Read the model definition and answer for the solid it produces. Units are mm, in the model's axes. Face numbers are marked on the shaded views. A direction names the side the tool comes from. Coordinates: 2 decimals unless noted, no trailing zeros. Order: outer loops, then holes, each group sorted by start corner. A loop starts at its lowest first (then second) coordinate and runs counter-clockwise, first axis right, second up. Notation, with made-up numbers: M 26,21.5 L 33,21.5 A10 ccw 33,29.5 Z; hole C 10,49 d7. An arc over 180 degrees is marked long. Put each result on its own line as item: value.
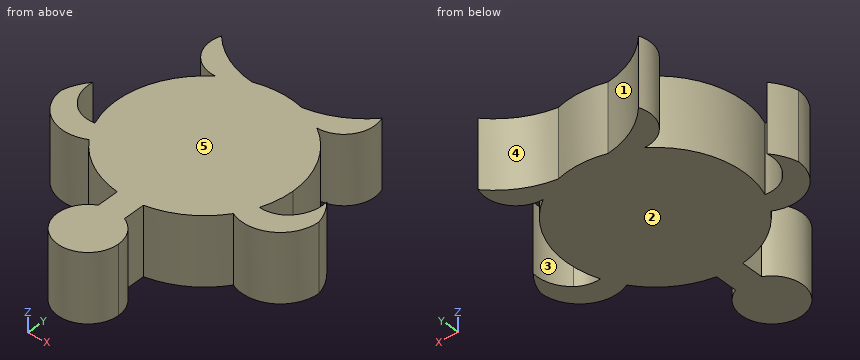
from build123d import *

# Parameters (mm, degrees)
F1_DEPTH = 2


with BuildPart() as f1:
    # F0 (on Top) → F1 (new body)
    with BuildSketch(Plane.XY):
        with BuildLine():
            ThreePointArc((-1.484384, 2.124211), (-1.120709, 2.336596), (-0.727436, 2.487269))
            ThreePointArc((-0.727436, 2.487269), (-1.616601, 2.768638), (-2.351094, 3.343359))
            ThreePointArc((-2.351094, 3.343359), (-2.243244, 2.502379), (-1.484384, 2.124211))
        make_face()
        with BuildLine():
            ThreePointArc((-2.113658, -1.499373), (-2.279864, -1.232027), (-2.412428, -0.9465))
            ThreePointArc((-2.412428, -0.9465), (-2.750971, -0.923594), (-3.055104, -0.773129))
            ThreePointArc((-3.055104, -0.773129), (-3.36643, -0.345932), (-3.426473, 0.17925))
            ThreePointArc((-3.426473, 0.17925), (-3.640466, -0.140011), (-3.772722, -0.500882))
            ThreePointArc((-3.772722, -0.500882), (-3.219918, -1.459931), (-2.113658, -1.499373))
        make_face()
        with BuildLine():
            ThreePointArc((3.055104, -0.773129), (2.750971, -0.923594), (2.412428, -0.9465))
            ThreePointArc((2.412428, -0.9465), (2.279864, -1.232027), (2.113658, -1.499373))
            ThreePointArc((2.113658, -1.499373), (3.219918, -1.459931), (3.772722, -0.500882))
            ThreePointArc((3.772722, -0.500882), (3.640466, -0.140011), (3.426473, 0.17925))
            ThreePointArc((3.426473, 0.17925), (3.36643, -0.345932), (3.055104, -0.773129))
        make_face()
        with BuildLine():
            ThreePointArc((0.892009, -4.021506), (0.754487, -3.54566), (0.384325, -3.216537))
            ThreePointArc((0.384325, -3.216537), (0, -3.129497), (-0.384325, -3.216537))
            ThreePointArc((-0.384325, -3.216537), (-0.475846, -4.775993), (0.892009, -4.021506))
        make_face()
        with BuildLine():
            ThreePointArc((2.591461, 0), (2.298085, 1.197695), (1.484384, 2.124211))
            ThreePointArc((1.484384, 2.124211), (1.120709, 2.336596), (0.727436, 2.487269))
            ThreePointArc((0.727436, 2.487269), (0, 2.591461), (-0.727436, 2.487269))
            ThreePointArc((-0.727436, 2.487269), (-1.120709, 2.336596), (-1.484384, 2.124211))
            ThreePointArc((-1.484384, 2.124211), (-2.480645, 0.749711), (-2.412428, -0.9465))
            ThreePointArc((-2.412428, -0.9465), (-2.276223, -1.230181), (-2.111146, -1.498092))
            ThreePointArc((-2.111146, -1.498092), (-2.112401, -1.498733), (-2.113658, -1.499373))
            ThreePointArc((-2.113658, -1.499373), (-1.357461, -2.20748), (-0.384325, -2.562804))
            ThreePointArc((-0.384325, -2.562804), (0, -2.591461), (0.384325, -2.562804))
            ThreePointArc((0.384325, -2.562804), (1.357461, -2.20748), (2.113658, -1.499373))
            ThreePointArc((2.113658, -1.499373), (2.279864, -1.232027), (2.412428, -0.9465))
            ThreePointArc((2.412428, -0.9465), (2.546309, -0.481642), (2.591461, 0))
        make_face()
        with BuildLine():
            ThreePointArc((0.727436, 2.487269), (1.120709, 2.336596), (1.484384, 2.124211))
            ThreePointArc((1.484384, 2.124211), (2.243244, 2.502379), (2.351094, 3.343359))
            ThreePointArc((2.351094, 3.343359), (1.616601, 2.768638), (0.727436, 2.487269))
        make_face()
        with BuildLine():
            Line((0.384325, -3.216537), (0.384325, -2.562804))
            ThreePointArc((0.384325, -2.562804), (0, -2.591461), (-0.384325, -2.562804))
            Line((-0.384325, -2.562804), (-0.384325, -3.216537))
            ThreePointArc((-0.384325, -3.216537), (0, -3.129497), (0.384325, -3.216537))
        make_face()
        with BuildLine():
            ThreePointArc((-2.111146, -1.498092), (-2.276223, -1.230181), (-2.412428, -0.9465))
            ThreePointArc((-2.412428, -0.9465), (-2.279864, -1.232027), (-2.113658, -1.499373))
            ThreePointArc((-2.113658, -1.499373), (-2.112401, -1.498733), (-2.111146, -1.498092))
        make_face()
    extrude(amount=F1_DEPTH)


solid = f1.part
Q1. Consider line 1 along Y through (x, z) = (0, 0.6); line 2 along X through (y, z) = (-0.5, 1.3); line 3 along Y through (x, z) = (-1.75, 1.6). Determine where each line is inside the solid, lowest interval first.
Answers below:
line 1: y = -4.91 to 2.59
line 2: x = -3.77 to -3.29, -2.54 to 2.54, 3.29 to 3.77
line 3: y = -1.91 to 1.91, 2.16 to 2.84
Q2. A tool of negligible diameter and unlimited length cuts with its end or side. For the marked faces 1, 2 and 3, from which of +Z, -Z, +X, -X, +Y, -Y can it reach the whole face along a straight path? Write none if from no direction.
Answers below:
face 1: +Z, -Z, +Y
face 2: -Z, +X, -X, +Y, -Y
face 3: +Z, -Z
Q3. Given pin 1 (0.7 mm diameter, centred on y = -3, z = 1, fed in from -X), flat-ended and moving along its own axis, determine where the tip first touches the part or whether it passes through.
Answers below:
pin 1: stops at x = -0.59
Q4. Find section C-C on x = 0. Write down the section's boundary in (y, z).
Answers below:
outline: M -4.91,0 L 2.59,0 L 2.59,2 L -4.91,2 Z
Q5. For a pull along X with two mould halves and no side action, classify the marked faces 4 and 5 as +X half, -X half, draft (parallel to the pull), parting line (faces both ways), or undercut.
Answers below:
face 4: undercut
face 5: draft
Q6. Find section A-A on y = 2.75. Write down the section's boundary in (x, z), plus the area to 3 significant figures.
Answers below:
outline: M -2.37,0 L -1.58,0 L -1.58,2 L -2.37,2 Z; M 1.58,0 L 2.37,0 L 2.37,2 L 1.58,2 Z
area: 3.15 mm^2
Q7. Find section B-B on z = 0.55. Write down the section's boundary in (x, y), plus the area to 3 significant figures.
Answers below:
outline: M -3.77,-0.5 A1.14 ccw -2.11,-1.5 A2.59 ccw -0.38,-2.56 L -0.38,-3.22 A0.89 ccw long 0.89,-4.02 A0.89 ccw 0.38,-3.22 L 0.38,-2.56 A2.59 ccw 2.11,-1.5 A1.14 ccw 3.77,-0.5 A1.61 ccw 3.43,0.18 A1.04 cw 3.06,-0.77 A0.87 cw 2.41,-0.95 A2.59 ccw 2.59,0 A2.59 ccw 1.48,2.12 A0.9 ccw 2.35,3.34 A2.62 cw 0.73,2.49 A2.59 ccw -0.73,2.49 A2.62 cw -2.35,3.34 A0.9 ccw -1.48,2.12 A2.59 ccw -2.41,-0.95 A0.87 cw -3.06,-0.77 A1.04 cw -3.43,0.18 A1.61 ccw Z
area: 28.1 mm^2
Q8. Find section D-D on y = -1.25. Write down the section's boundary in (x, z), plus the area to 3 significant figures.
Answers below:
outline: M -3.48,0 L 3.48,0 L 3.48,2 L -3.48,2 Z
area: 13.9 mm^2
